Build history of the part. All positions in model axes, mm. Give positions to 0.01 mm unless a question says otherwise; leave off trailing zeros. Loops run counter-clockwise (first coordinate to the right, second up) from the corner with the lowest first, then second, coordinate; pieces in that order, holes last. Notation, with made-up numbers: M -30.75,34 L 3.25,34 A21 cw 3.25,66 Z; hole C -40,57.5 d10. An arc over 180 degrees is marked long. Answer as a JSON object with one key per item and string values. Group by question number.
1. Drill centre lines: line 1 along Z through (x, y) = (11.75, 0); line 2 along Z through (x, y) = (-3, 19); line 3 along Y through (x, z) = (6, 26.5). Where is each one in solid material? Low to high. Write a range as [from, to].
2. Slice it at A-A (z = 0). List the corners of the cut face in (x, y), then the cut area to 3 significant figures.
3. Drop flat-ended pins along their axis: pin 1 Ø1.5 at (x, z) = (-4, -9) entering from +Y; pin 2 Ø2 at (x, y) = (-3.5, 12.5) entering from -Z; pin 3 Ø3 at (x, z) = (8, 8.5) entering from -Y. Give the stop position or say it passes through.
4. Slice it at C-C (x = 4). List the corners of the cut face in (y, z).
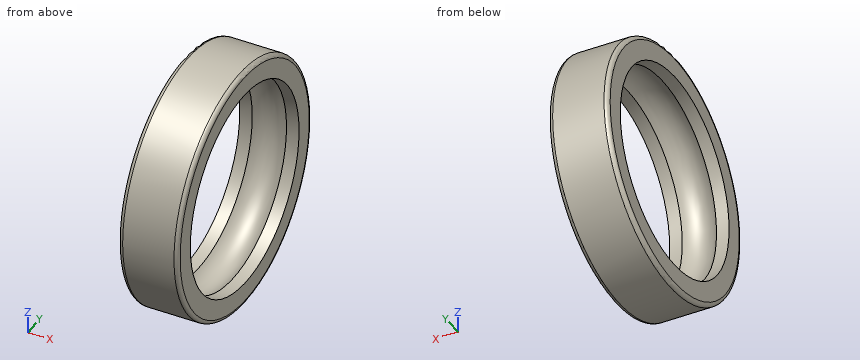
from build123d import *

# Parameters (mm, degrees)
FILLET1_R = 2.1


with BuildPart() as part:
    # Sketch3 → Revolve1 (revolve)
    with BuildSketch(Plane.XY):
        with BuildLine():
            Line((-15.339778092, 53), (-8.784050002, 53))
            ThreePointArc((-8.784050002, 53), (0.160221908, 57), (9.104493818, 53))
            Line((9.104493818, 53), (15.660221908, 53))
            Line((15.660221908, 53), (15.660221908, 65))
            Line((15.660221908, 65), (-15.339778092, 65))
            Line((-15.339778092, 65), (-15.339778092, 53))
        make_face()
    revolve(axis=Axis((-16.039993209, 0, 0), (1, 0, 0)))

    # Fillet1
    fillet1_edges = [part.edges().sort_by_distance(p)[0] for p in [
        (15.660221908, -65, 0),
        (-15.339778092, -65, 0),
    ]]
    fillet(fillet1_edges, radius=FILLET1_R)


solid = part.part
Established:
{
 "1": {"line 1": "z = [-65, -53], [53, 65]", "line 2": "z = [-62.16, -53.29], [53.29, 62.16]", "line 3": "y = [-59.35, -48.75], [48.75, 59.35]"},
 "2": {"outline": "M -15.34,-62.9 A2.1 ccw -13.24,-65 L 13.56,-65 A2.1 ccw 15.66,-62.9 L 15.66,-53 L 9.1,-53 A12 cw -8.78,-53 L -15.34,-53 Z; M -15.34,53 L -8.78,53 A12 cw 9.1,53 L 15.66,53 L 15.66,62.9 A2.1 ccw 13.56,65 L -13.24,65 A2.1 ccw -15.34,62.9 Z", "area": "641 mm^2"},
 "3": {"pin 1": "stops at y = 64.47", "pin 2": "stops at z = -63.97", "pin 3": "stops at y = -64.62"},
 "4": {"outline": "C 0,0 d130; hole C 0,0 d112.74"}
}
